from build123d import *

# Parameters (mm, degrees)
SKETCH_1_R          = 20
SKETCH_2_R          = 12.5
FILLET_1_R          = 1
SKETCH_3_R          = 1.7
CUT_EXTRUDE_1_DEPTH = 29.670542506
CUT_EXTRUDE_2_DEPTH = 29.670542541
SKETCH_6_R          = 3
CUT_EXTRUDE_3_DEPTH = 5
CUT_EXTRUDE_4_DEPTH = 5


with BuildPart() as part:
    # 草图1 → 放样1 section 0
    with BuildSketch(Plane.XY):
        Circle(SKETCH_1_R)
    # 草图2 → 放样1 section 1
    with BuildSketch(Plane.XY.offset(10)):
        Circle(SKETCH_2_R)
    loft()

    # 圆角1
    fillet_1_edges = [part.edges().sort_by_distance(p)[0] for p in [
        (-12.5, 0, 10),
        (-20, 0, 0),
    ]]
    fillet(fillet_1_edges, radius=FILLET_1_R)

    # 草图3 → 切除-拉伸1 (cut, through all)
    with BuildSketch(Plane(origin=(0, 0, 0), x_dir=(-1, 0, 0), z_dir=(0, 0, -1))):
        with Locations((0, -14)):
            Circle(SKETCH_3_R)
        with Locations((-12.124355653, 7)):
            Circle(SKETCH_3_R)
        with Locations((12.124355653, 7)):
            Circle(SKETCH_3_R)
        with Locations((0, 8.75)):
            Circle(SKETCH_3_R)
        with Locations((7.577722283, -4.375)):
            Circle(SKETCH_3_R)
        with Locations((-7.577722283, -4.375)):
            Circle(SKETCH_3_R)
    extrude(amount=-CUT_EXTRUDE_1_DEPTH, mode=Mode.SUBTRACT)

    # 草图5 → 切除-拉伸2 (cut, through all)
    with BuildSketch(Plane(origin=(0, 0, 0), x_dir=(-1, 0, 0), z_dir=(0, 0, -1))):
        Polygon((-3, 5.196152423), (-6, 0), (-3, -5.196152423), (3, -5.196152423), (6, 0), (3, 5.196152423), align=None)
    extrude(amount=-CUT_EXTRUDE_2_DEPTH, mode=Mode.SUBTRACT)

    # 草图6 → 切除-拉伸3 (cut)
    with BuildSketch(Plane(origin=(0, 0, 0), x_dir=(-1, 0, 0), z_dir=(0, 0, -1))):
        with Locations((-7.577722283, -4.375)):
            Circle(SKETCH_6_R)
        with Locations((7.577722283, -4.375)):
            Circle(SKETCH_6_R)
        with Locations((0, 8.75)):
            Circle(SKETCH_6_R)
    extrude(amount=-CUT_EXTRUDE_3_DEPTH, mode=Mode.SUBTRACT)

    # 草图7 → 切除-拉伸4 (cut)
    with BuildSketch(Plane.XY.offset(10)):
        Polygon((-15.624355653, 7), (-13.874355653, 3.968911087), (-10.374355653, 3.968911087), (-8.624355653, 7), (-10.374355653, 10.031088913), (-13.874355653, 10.031088913), align=None)
        Polygon((13.874355653, 3.968911087), (15.624355653, 7), (13.874355653, 10.031088913), (10.374355653, 10.031088913), (8.624355653, 7), (10.374355653, 3.968911087), align=None)
        Polygon((-1.75, -10.968911087), (-3.5, -14), (-1.75, -17.031088913), (1.75, -17.031088913), (3.5, -14), (1.75, -10.968911087), align=None)
    extrude(amount=-CUT_EXTRUDE_4_DEPTH, mode=Mode.SUBTRACT)


solid = part.part
Work out the finished part from the listing and answer in its coordinate system (mm). A direction names the side the tool comes from. Give positions to 0.01 mm unless a question says otherwise; leave off trailing zeros. Loops run counter-clockwise (first coordinate to the right, second up) from the corner with the lowest first, then second, coordinate; pieces in that order, holes last. Notation, with made-up numbers: (26.25, 72.25) - (59.25, 72.25) arc R5 cw to (59.25, 79.25) - close; hole circle Ø1 at (-14.75, -26). An arc over 180 degrees is marked (long way). Answer in a Markdown table with one row per item.
(1) Consider L1, parallel to Y at x = 1, z = 3; L2, parallel to X at y = -5.5, z = 6; L3, parallel to Y at x = 0, z = 1.7 (3 decimals). Determine where each line is inside the solid, lowest interval first. Write a range as [from, to].
Results list:
| item | result |
|---|---|
| L1 | y = [-17.72, -15.37], [-12.63, -5.2], [5.2, 5.92], [11.58, 17.72] |
| L2 | x = [-14.49, -8.85], [-6.3, 6.3], [8.85, 14.49] |
| L3 | y = [-18.725, -15.7], [-12.3, -5.196], [5.196, 5.75], [11.75, 18.725] |
(2) Section A-A (x = 0) is taken. Give the vertices of the cut face in (y, z), and give its area (3 significant figures).
Results list:
| item | result |
|---|---|
| outline | (-18.8, 1.6) arc R1 ccw to (-18, 0) - (-15.7, 0) - (-15.7, 5) - (-16.25, 5) - close; (-12.3, 0) - (-5.2, 0) - (-5.2, 10) - (-10.97, 10) - (-10.97, 5) - (-12.3, 5) - close; (5.2, 0) - (5.75, 0) - (5.75, 5) - (7.05, 5) - (7.05, 10) - (5.2, 10) - close; (10.45, 5) - (11.75, 5) - (11.75, 0) - (18, 0) arc R1 ccw to (18.8, 1.6) - (12.8, 9.6) arc R1 ccw to (12, 10) - (10.45, 10) - close |
| area | 138 mm² |
(3) Flat-ended cylindrical pins translate along their axes: pin 1 Ø3 at (x, y) = (0, 10) entering from -Z; pin 2 Ø1.8 at (x, z) = (-12.5, 7) entering from +Y; pin 3 Ø1.9 at (x, z) = (-12, 5.5) entering from -Y. Find the tip coordinate at first contact, or state that the pin passes through.
Results list:
| item | result |
|---|---|
| pin 1 | stops at z = 5 |
| pin 2 | stops at y = 3.97 |
| pin 3 | stops at y = -11.83 |
(4) Section B-B (z = 6.75) is taken. State how many separate pieces and enclosed holes the cut face has, and give its area (3 significant figures).
Results list:
| item | result |
|---|---|
| separate pieces | 1 |
| enclosed holes | 4 |
| area | 516 mm² |
(5) A tool of negligible diameter and unlimited length cuts with its end or side. For faces 1 (the face through (11, 10.031, 6)), 2 (the face through (4.5, -2.6, 4.9)), 3 (the face through (-11, 10.031, 6)), 4 (the face through (-2.61, -12.46, 6.98)), from which of +Z, -Z, +X, -X, +Y, -Y can it reach the whole face along a straight path? Write none if from no direction.
Results list:
| item | result |
|---|---|
| face 1 | +Z, +X |
| face 2 | +Z, -Z |
| face 3 | +Z, -X |
| face 4 | +Z |
(6) For a pull along Y with two mould halves and no side action, classify faces 5 (the face through (-14.218, 4.563, 5.691)), 6 (the face through (0, -10.969, 8)), 7 (the face through (4.5, 2.6, 4.9)) as pulls with the +Y half, pulls with the -Y half, needs draft (parallel to the pull), parting line crosses it, or undercut.
Results list:
| item | result |
|---|---|
| face 5 | pulls with the +Y half |
| face 6 | pulls with the -Y half |
| face 7 | undercut |
(7) Section C-C (z = 2.5) is taken. Give the vertices of the cut face in (x, y) (3 decimals).
Results list:
| item | result |
|---|---|
| outline | circle Ø36.25 at (0, 0); hole circle Ø3.4 at (-12.124, 7); hole circle Ø6 at (-7.578, -4.375); hole (-6, 0) - (-3, -5.196) - (3, -5.196) - (6, 0) - (3, 5.196) - (-3, 5.196) - close; hole circle Ø6 at (0, 8.75); hole circle Ø3.4 at (0, -14); hole circle Ø6 at (7.578, -4.375); hole circle Ø3.4 at (12.124, 7) |
